Autodesk Inventor part; units mm, degrees
ref_plane "YZ Plane" through (0, 0, 0) normal (1, 0, 0) x (0, 1, 0)
ref_plane "XZ Plane" through (0, 0, 0) normal (0, 1, 0) x (-1, 0, 0)
ref_plane "XY Plane" through (0, 0, 0) normal (0, 0, 1) x (1, 0, 0)
sketch "Sketch1" plane through (0, 0, 0) normal (0, 1, 0) x (-1, 0, 0)
  line L0 (0, 0) -> (203.2, 0)
  line L1 (203.2, 0) -> (203.2, -68.58)
  line L2 (203.2, -68.58) -> (0, -68.58)
  line L3 (0, -68.58) -> (0, 0)
  dimension "d0" = 203.2
  dimension "d1" = 68.58
extrude "Extrusion1" add sketch "Sketch1" along normal blind 6.35
sketch "Sketch2" plane through (0, 6.35, 0) normal (0, 1, 0) x (1, 0, 0)
  line L0 (-184.15, 0) -> (-190.5, 0)
  line L1 (-190.5, 0) -> (-190.5, -12.7)
  line L2 (-190.5, -12.7) -> (-184.15, -12.7)
  line L3 (-184.15, -12.7) -> (-184.15, 0)
  circle A0 centre (-187.325, -9.525) radius 1.397
  line L4 (-203.2, 0) -> (0, 0)
  line L5 (-22.225, 0) -> (-28.575, 0)
  line L6 (-28.575, 0) -> (-28.575, -12.7)
  line L7 (-28.575, -12.7) -> (-22.225, -12.7)
  line L8 (-22.225, -12.7) -> (-22.225, 0)
  circle A1 centre (-25.4, -9.525) radius 1.397
  dimension "d4" = 12.7
  dimension "d5" = 6.35
  dimension "d6" = 2.794
  dimension "d7" = 3.175
  dimension "d8" = 3.175
  dimension "d9" = 0
  dimension "d10" = 12.7
  dimension "d11" = 12.7
  dimension "d12" = 6.35
  dimension "d13" = 2.794
  dimension "d14" = 3.175
  dimension "d15" = 3.175
  dimension "d16" = 0
  dimension "d20" = 25.4
extrude "Extrusion2" add sketch "Sketch2" against normal blind 6.35
ref_plane "Work Plane1" through (-184.15, 0, -34.29) normal (0, 0, 1) x (1, 0, 0)
mirror "Mirror1" about plane through (-184.15, 0, -34.29) normal (0, 0, 1) of "Extrusion2"
sketch "Sketch3" plane through (0, 6.35, 0) normal (0, 1, 0) x (1, 0, 0)
  line L0 (-156.845, 41.91) -> (-100.965, 41.91)
  line L1 (-100.965, 41.91) -> (-100.965, 60.96)
  line L2 (-100.965, 60.96) -> (-156.845, 60.96)
  line L3 (-156.845, 60.96) -> (-156.845, 41.91)
  line L4 (-156.845, 41.91) -> (-139.065, 41.91)
  line L5 (-139.065, 41.91) -> (-139.065, 24.13)
  line L6 (-139.065, 24.13) -> (-156.845, 24.13)
  line L7 (-156.845, 24.13) -> (-156.845, 41.91)
  line L8 (-28.575, 68.58) -> (-184.15, 68.58)
  circle A0 centre (-187.325, 78.105) radius 1.397
  point P0 (0, 0)
  dimension "d21" = 19.05
  dimension "d22" = 55.88
  dimension "d23" = 17.78
  dimension "d24" = 17.78
  dimension "d25" = 7.62
  dimension "d28" = 30.48
extrude "Extrusion3" cut sketch "Sketch3" against normal blind 25.4 contours L3 L2 L1 L0 | L0 L5 L6 L7
properties part number "BackPanel"
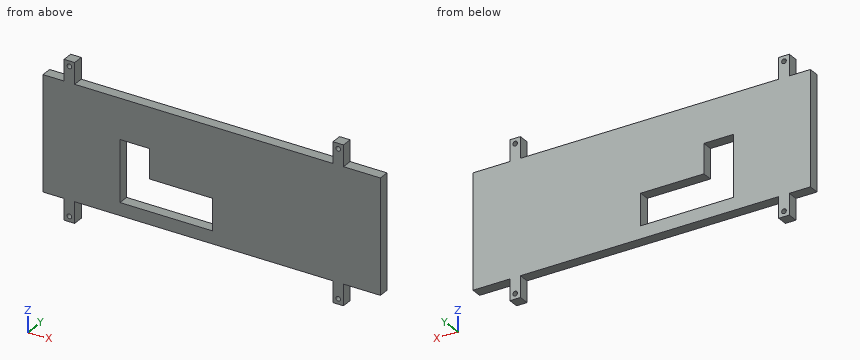
Build history of the part. All positions in model axes, mm. Round coordinates to 2 decimals unless told otherwise and drop trailing zeros. Loops run counter-clockwise (first coordinate to the right, second up) from the corner with the lowest first, then second, coordinate; pieces in that order, holes last.
Item 1: Pin check, flat tips, straight feed: P1, Ø1.5, axis at x = -172.5, y = 2, coming from the -Z side; P2, Ø1, axis at x = -61, y = 1.5, coming from the +Z side; P3, Ø1.9, axis at y = 3.5, z = 6, coming from the -X side. Stop position of each tip, or through.
Item 2: Saw through at C-C (x = -67). List the corners of the cut face in (y, z).
Item 3: Saw through at B-B (y = 4.75). State how many separate pieces and enclosed holes the cut face has, then the cut area to 3 significant figures.
Item 4: Saw through at A-A (z = 3.5). List the corners of the cut face in (x, y) (3 decimals).
Item 5: Drill centre lines: line 1 along Z through (x, y) = (-25.4, 5); line 2 along Z through (x, y) = (-107.5, 2.5); line 3 along X through (y, z) = (4.75, 2) (3 decimals). Where is each one in solid material? Low to high.
Worked answers:
1. P1: stops at z = -68.58
1. P2: stops at z = 0
1. P3: stops at x = -190.5
2. outline: (0, -68.58) - (6.35, -68.58) - (6.35, 0) - (0, 0) - close
3. separate pieces: 1
3. enclosed holes: 5
3. area: 12,900 mm2
4. outline: (-190.5, 0) - (-184.15, 0) - (-184.15, 6.35) - (-190.5, 6.35) - close; (-28.575, 0) - (-22.225, 0) - (-22.225, 6.35) - (-28.575, 6.35) - close
5. line 1: z = -81.28 to -79.5, -76.71 to 8.13, 10.92 to 12.7
5. line 2: z = -68.58 to -60.96, -41.91 to 0
5. line 3: x = -190.5 to -184.15, -28.575 to -22.225
